```python
from build123d import *

# Parameters (mm, degrees)
BOSS_EXTRUDE1_DEPTH = 18
BOSS_EXTRUDE2_DEPTH = 1


with BuildPart() as part:
    # Sketch1 → Boss-Extrude1 (new body)
    with BuildSketch(Plane(origin=(0, 0, 0), x_dir=(1, 0, 0), z_dir=(0, 1, 0))):
        with BuildLine():
            ThreePointArc((30.88932948, 3), (26.70932948, 7.18), (22.52932948, 3))
            Line((22.52932948, 3), (22.52932948, 0))
            Line((22.52932948, 0), (22.52932948, -0.2))
            Line((22.52932948, -0.2), (22.72932948, -0.2))
            Line((22.72932948, -0.2), (22.72932948, 0))
            Line((22.72932948, 0), (22.72932948, 3))
            ThreePointArc((22.72932948, 3), (26.70932948, 6.98), (30.68932948, 3))
            Line((30.68932948, 3), (30.68932948, 0))
            Line((30.68932948, 0), (30.68932948, -0.2))
            Line((30.68932948, -0.2), (30.88932948, -0.2))
            Line((30.88932948, -0.2), (30.88932948, 0))
            Line((30.88932948, 0), (30.88932948, 3))
        make_face()
    extrude(amount=BOSS_EXTRUDE1_DEPTH)

    # Sketch1_4 → Boss-Extrude2 (add)
    with BuildSketch(Plane(origin=(0, 0, 0), x_dir=(1, 0, 0), z_dir=(0, 1, 0))):
        with BuildLine():
            ThreePointArc((30.88932948, 3), (26.70932948, 7.18), (22.52932948, 3))
            Line((22.52932948, 3), (22.52932948, 0))
            Line((22.52932948, 0), (22.52932948, -0.2))
            Line((22.52932948, -0.2), (22.72932948, -0.2))
            Line((22.72932948, -0.2), (22.72932948, 0))
            Line((22.72932948, 0), (22.72932948, 3))
            ThreePointArc((22.72932948, 3), (26.70932948, 6.98), (30.68932948, 3))
            Line((30.68932948, 3), (30.68932948, 0))
            Line((30.68932948, 0), (30.68932948, -0.2))
            Line((30.68932948, -0.2), (30.88932948, -0.2))
            Line((30.88932948, -0.2), (30.88932948, 0))
            Line((30.88932948, 0), (30.88932948, 3))
        make_face()
    extrude(amount=-BOSS_EXTRUDE2_DEPTH)


solid = part.part
```
Design review of the part built by this model. Coordinates are the model's own, in mm. A direction names the side the tool comes from. Coordinates: 2 decimals unless noted, no trailing zeros. Order: outer loops, then holes, each group sorted by start corner. A loop starts at its lowest first (then second) coordinate and runs counter-clockwise, first axis right, second up. Notation, with made-up numbers: M -18.75,76 L 34.25,76 A26 ccw 34.25,104 Z; hole C 54.25,-7.5 d1. An arc over 180 degrees is marked long. Answer as a JSON object with one key per item and string values. Group by question number.
1) Tool access review of faces 1 (the flat face through (30.689, 9, -1)), 2 (the cylindrical face through (26.8, 8.63, -7.18)): name each direction out of +Z, -Z, +X, -X, +Y, -Y from which nothing blocks a thin tool from reaching the whole face with its end or side.
2) Add section A-A, the plane z = -1.5. Write out the cut boundary in (x, y).
3) Add section C-C, the plane z = -6.25. Write out the cut boundary in (x, y).
4) Add section B-B, the plane y = 13.5. Write out the cut boundary in (x, z).
5) Add section D-D, the plane x = 28.25. Write out the cut boundary in (y, z).
6) Mouldability with a two-part tool opening along X and no side actions: class faces 3 (the flat face through (22.529, 9, -1)), 4 (the flat face through (30.889, 9, -1)), 5 (the cylindrical face through (26.62, 8.63, -6.98)), 6 (the flat face through (22.729, 9, -1)) as pulls with the +X half, pulls with the -X half, needs draft (parallel to the pull), parting line crosses it, or undercut.
7) For pin 1 (1 mm diameter, centred on x = 29, y = 5, fed in from +Z); pin 2 (3 mm diameter, centred on x = 28, z = -6, fed in from -Y); pin 3 (1.5 mm diameter, centred on y = 10, z = -5.5, fed in from +X); pin 4 (1 mm diameter, centred on y = 2, z = -5, fed in from +X), all flat-tipped, find the tip position at first contact; note any pin that passes through.
8) Wall thickness on L1, parallel to X at y = 2.5, z = -2.5; L2, parallel to X at y = 1.5, z = -5; L3, parallel to Z at x = 26, y = 6.5: over which ranges is each line inside the solid? List them lowest first.
Computed values:
{
 "1": {"face 1": "+Z, +Y, -Y", "face 2": "-Z, +Y, -Y"},
 "2": {"outline": "M 22.53,-1 L 22.73,-1 L 22.73,18 L 22.53,18 Z; M 30.69,-1 L 30.89,-1 L 30.89,18 L 30.69,18 Z"},
 "3": {"outline": "M 24.08,-1 L 24.41,-1 L 24.41,18 L 24.08,18 Z; M 29.01,-1 L 29.34,-1 L 29.34,18 L 29.01,18 Z"},
 "4": {"outline": "M 22.53,-3 A4.18 ccw 30.89,-3 L 30.89,0.2 L 30.69,0.2 L 30.69,-3 A3.98 cw 22.73,-3 L 22.73,0.2 L 22.53,0.2 Z"},
 "5": {"outline": "M -1,-6.89 L 18,-6.89 L 18,-6.67 L -1,-6.67 Z"},
 "6": {"face 3": "pulls with the -X half", "face 4": "pulls with the +X half", "face 5": "undercut", "face 6": "undercut"},
 "7": {"pin 1": "stops at z = -5.84", "pin 2": "stops at y = -1", "pin 3": "stops at x = 30.51", "pin 4": "stops at x = 30.61"},
 "8": {"L1": "x = 22.53 to 22.73, 30.69 to 30.89", "L2": "x = 23.04 to 23.27, 30.15 to 30.38", "L3": "z = -7.12 to -6.92"}
}
